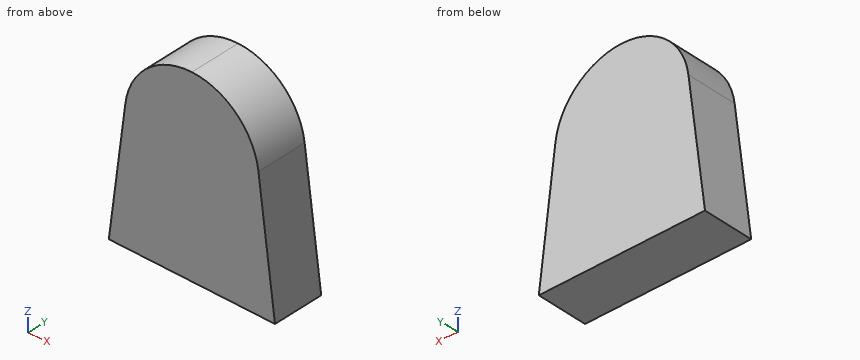
Autodesk Inventor part; units mm, degrees
ref_plane "YZ Plane" through (0, 0, 0) normal (1, 0, 0) x (0, 1, 0)
ref_plane "XZ Plane" through (0, 0, 0) normal (0, 1, 0) x (-1, 0, 0)
ref_plane "XY Plane" through (0, 0, 0) normal (0, 0, 1) x (1, 0, 0)
sketch "Skizze1" plane through (0, 0, 0) normal (0, 1, 0) x (-1, 0, 0)
  arc A0 (12.3985, 1.5897) -> (0, 12.5) centre (0, 0) ccw
  line L0 (0, -34.7678) -> (0, 23.1071) construction
  line L1 (12.3985, 1.5897) -> (16, -26.5)
  line L2 (16, -26.5) -> (0, -26.5)
  arc A1 (0, 12.5) -> (-12.3985, 1.5897) centre (0, 0) ccw
  line L3 (-12.3985, 1.5897) -> (-16, -26.5)
  line L4 (-16, -26.5) -> (0, -26.5)
  line L5 (15.4871, -22.5) -> (-15.4871, -22.5)
  dimension "d0" = 25
  dimension "d1" = 32
  dimension "d2" = 39
  dimension "d3" = 35
extrude "Extrusion1" add sketch "Skizze1" along normal blind 9.5 contours L1 L5 L3 A1 A0
properties part number "Steitenteil_voll"
CAD build for the part. Positions are in the model's coordinates, mm. Round coordinates to 2 decimals unless told otherwise and drop trailing zeros. Write each loop counter-clockwise with the first axis right and the second up, starting at its lowest first coordinate (ties: lowest second). Pieces come first, ordered by that corner, then holes. Notation, with made-up numbers: (-14, 76.5) -> (19, 76.5) arc R22 cw to (19, 95.5) -> close; hole circle Ø1 at (89.5, -10). An arc over 180 degrees is marked (long way). Answer in a Markdown table with one row per item. Add a question column.
Item 1: Saw through at C-C, the plane x = -8. Write the cut outline in (y, z).
Item 2: Drill centre lines: line 1 (X direction, y = 5.75, z = -5); line 2 (X direction, y = 1, z = -7); line 3 (Z direction, x = 8.5, y = 6.5). Where is each one in solid material? Low to high. Write a range as from..to.
Item 3: Saw through at A-A, the plane y = 3.5. Write the cut outline in (x, z), then the cut area to 3 significant figures.
Item 4: Drop flat-ended pins along their axis: pin 1 Ø1.5 at (x, y) = (6.5, 8) entering from +Z; pin 2 Ø3 at (y, z) = (7, 7) entering from +X (3 decimals). Give the stop position or say it passes through.
Item 5: Saw through at B-B, the plane z = 6.5. Write the cut outline in (x, y).
Findings below:
| question | item | result |
|---|---|---|
| 1 | outline | (0, -22.5) -> (9.5, -22.5) -> (9.5, 9.6) -> (0, 9.6) -> close |
| 2 | line 1 | x = -13.24..13.24 |
| 2 | line 2 | x = -13.5..13.5 |
| 2 | line 3 | z = -22.5..9.17 |
| 3 | outline | (-15.49, -22.5) -> (15.49, -22.5) -> (12.4, 1.59) arc R12.5 ccw to (0, 12.5) arc R12.5 ccw to (-12.4, 1.59) -> close |
| 3 | area | 878 mm^2 |
| 4 | pin 1 | stops at z = 11.1 |
| 4 | pin 2 | stops at x = 11.225 |
| 5 | outline | (-10.68, 0) -> (10.68, 0) -> (10.68, 9.5) -> (-10.68, 9.5) -> close |
